Part model, mm, in its own coordinate system. Face numbers are marked on the shaded views. Give positions to 0.01 mm unless a question says otherwise; leave off trailing zeros. Write each loop counter-clockwise with the first axis right and the second up, starting at its lowest first coordinate (ties: lowest second). Pieces come first, ordered by that corner, then holes. Notation, with made-up numbers: (0, 31) - (47, 31) arc R7 ccw to (47, 40) - close; hole circle Ø1 at (88, 5). An arc over 180 degrees is marked (long way). Answer in a Markdown table with one row per item. Add a question column.
1. Pull direction X, two halves, no side cores. Call the marked faces 1, 2, 3 and 4: released by +X, released by -X, zero draft, split by the parting line, or undercut.
2. Band-saw the part on B-B on x = -50. Write the cut outline in (y, z), plus the area to 3 significant figures.
3. Band-saw the part on A-A on y = 0. Write the cut outline in (x, z), plus the area to 3 significant figures.
4. Drop flat-ended pins along their axis: pin 1 Ø1 at (y, z) = (26.5, 5) entering from -X; pin 2 Ø10 at (x, y) = (-54.5, -5.5) entering from -Z; pin 3 Ø2 at (y, z) = (-21.5, 3.5) entering from -X. Give the stop position or say it passes through.
5. Band-saw the part on D-D on y = -24.5. Write the cut outline in (x, z), plus the area to 3 significant figures.
6. Band-saw the part on C-C on z = 6. Write the cut outline in (x, y), plus the area to 3 significant figures.
7. Probe line 1 along Y through (x, z) = (-63.5, 13.5); line 2 along X through (y, z) = (0, 20.25); line 3 along Y through (x, z) = (-67.5, 15). List the from-to ranges inside material, lowest first.
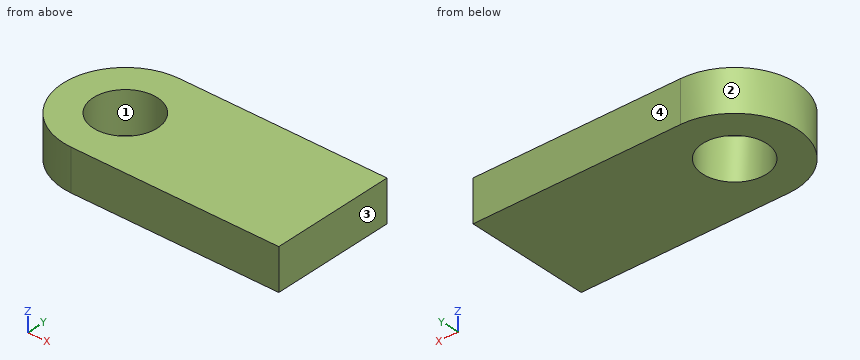
```python
from build123d import *

# Parameters (mm, degrees)
F1_DEPTH = 25.4
F2_DEPTH = 25.4
F3_DEPTH = 25.4


with BuildPart() as f1:
    # F0 (on Top) → F1 (new body)
    with BuildSketch(Plane.XY):
        with BuildLine():
            Line((-63.5, 19.565446079), (-63.5, -19.565446079))
            ThreePointArc((-63.5, -19.565446079), (-49.6651404006, -13.8348595994), (-43.934553921, 0))
            ThreePointArc((-43.934553921, 0), (-49.6651404006, 13.8348595994), (-63.5, 19.565446079))
        make_face()
        with BuildLine():
            ThreePointArc((-63.5, 19.565446079), (-83.065446079, 0), (-63.5, -19.565446079))
            Line((-63.5, -19.565446079), (-63.5, 19.565446079))
        make_face()
    extrude(amount=F1_DEPTH)

    # F0 (on Top) → F2 (join)
    with BuildSketch(Plane.XY):
        with BuildLine():
            Line((-63.5, -38.1), (63.5, -38.1))
            Line((63.5, -38.1), (63.5, 38.1))
            Line((63.5, 38.1), (-63.5, 38.1))
            ThreePointArc((-63.5, 38.1), (-36.5592316368, 26.9407683632), (-25.4, 0))
            ThreePointArc((-25.4, 0), (-36.5592316368, -26.9407683632), (-63.5, -38.1))
        make_face()
        with BuildLine():
            ThreePointArc((-63.5, 38.1), (-101.6, 0), (-63.5, -38.1))
            Line((-63.5, -38.1), (-63.5, -19.565446079))
            ThreePointArc((-63.5, -19.565446079), (-83.065446079, 0), (-63.5, 19.565446079))
            Line((-63.5, 19.565446079), (-63.5, 38.1))
        make_face()
        with BuildLine():
            Line((-63.5, -19.565446079), (-63.5, -38.1))
            ThreePointArc((-63.5, -38.1), (-36.5592316368, -26.9407683632), (-25.4, 0))
            ThreePointArc((-25.4, 0), (-36.5592316368, 26.9407683632), (-63.5, 38.1))
            Line((-63.5, 38.1), (-63.5, 19.565446079))
            ThreePointArc((-63.5, 19.565446079), (-49.6651404006, 13.8348595994), (-43.934553921, 0))
            ThreePointArc((-43.934553921, 0), (-49.6651404006, -13.8348595994), (-63.5, -19.565446079))
        make_face()
    extrude(amount=F2_DEPTH)

    # F0 (on Top) → F3 (cut)
    with BuildSketch(Plane.XY):
        with BuildLine():
            ThreePointArc((-63.5, 19.565446079), (-83.065446079, 0), (-63.5, -19.565446079))
            Line((-63.5, -19.565446079), (-63.5, 19.565446079))
        make_face()
        with BuildLine():
            Line((-63.5, 19.565446079), (-63.5, -19.565446079))
            ThreePointArc((-63.5, -19.565446079), (-49.6651404006, -13.8348595994), (-43.934553921, 0))
            ThreePointArc((-43.934553921, 0), (-49.6651404006, 13.8348595994), (-63.5, 19.565446079))
        make_face()
    extrude(amount=F3_DEPTH, mode=Mode.SUBTRACT)


solid = f1.part
```
Values:
| question | item | result |
|---|---|---|
| 1 | face 1 | undercut |
| 1 | face 2 | released by -X |
| 1 | face 3 | released by +X |
| 1 | face 4 | zero draft |
| 2 | outline | (-38.1, 0) - (-14.16, 0) - (-14.16, 25.4) - (-38.1, 25.4) - close; (14.16, 0) - (38.1, 0) - (38.1, 25.4) - (14.16, 25.4) - close |
| 2 | area | 1,220 mm² |
| 3 | outline | (-101.6, 0) - (-83.07, 0) - (-83.07, 25.4) - (-101.6, 25.4) - close; (-43.93, 0) - (63.5, 0) - (63.5, 25.4) - (-43.93, 25.4) - close |
| 3 | area | 3,200 mm² |
| 4 | pin 1 | stops at x = -91.35 |
| 4 | pin 2 | passes through |
| 4 | pin 3 | stops at x = -95.61 |
| 5 | outline | (-92.68, 0) - (63.5, 0) - (63.5, 25.4) - (-92.68, 25.4) - close |
| 5 | area | 3,970 mm² |
| 6 | outline | (-63.5, -38.1) - (63.5, -38.1) - (63.5, 38.1) - (-63.5, 38.1) arc R38.1 ccw to start; hole circle Ø39.13 at (-63.5, 0) |
| 6 | area | 10,800 mm² |
| 7 | line 1 | y = -38.1 to -19.57, 19.57 to 38.1 |
| 7 | line 2 | x = -101.6 to -83.07, -43.93 to 63.5 |
| 7 | line 3 | y = -37.89 to -19.15, 19.15 to 37.89 |
